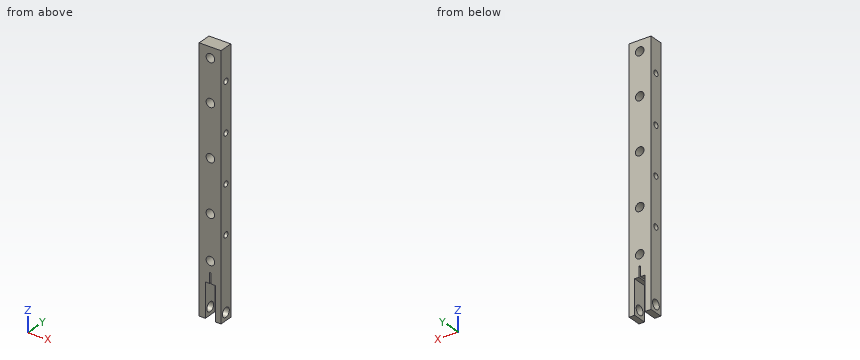
```python
from build123d import *

# Parameters (mm, degrees)
F1_DEPTH = 8
F3_D     = 5.5
F5_D     = 5
F7_D     = 3.3


with BuildPart() as f1:
    # F0 (on Front) → F1 (new body)
    with BuildSketch(Plane.XZ):
        Polygon((-6.6129033404, 0), (-3, 0), (-3, 20), (-0.5, 20), (-0.5, 26), (0.5, 26), (0.5, 20), (3, 20), (3, 0), (6.2258067564, 0), (6.2258067564, 150), (-6.6129033404, 150), align=None)
    extrude(amount=F1_DEPTH)

    # F3 (through all)
    with Locations(Plane(origin=(-6.6129033404, 0, 0), x_dir=(0, -1, 0), z_dir=(-1, 0, 0))):
        with Locations((4, 4.5417556539)):
            Hole(F3_D / 2)

    # F5 (through all)
    with Locations(Plane.XZ.offset(8)):
        with Locations((0, 32.4720963836), (0, 58.3593994379), (0, 88.90619874), (0, 119.1896349192), (0, 143.8203305006)):
            Hole(F5_D / 2)

    # F7 (through all)
    with Locations(Plane(origin=(-6.6129033404, 0, 0), x_dir=(0, -1, 0), z_dir=(-1, 0, 0))):
        with Locations((4, 131.3748806715), (4, 102.970726788), (4, 75), (4, 47.0387488604)):
            Hole(F7_D / 2)


solid = f1.part
```
Here's how the part is built. I have some questions about the finished solid (model axes, mm). Round coordinates to 2 decimals unless told otherwise and drop trailing zeros. Write each loop counter-clockwise with the first axis right and the second up, starting at its lowest first coordinate (ties: lowest second). Pieces come first, ordered by that corner, then holes.
Q1. If we section it at C-C on y = -4: Give the number of separate pieces and of enclosed holes in the cut face, plus the area to 3 significant figures.
Q2. Will this pin go through, and if not, where does the flat tip stop? P1, Ø0.8, axis at x = 2, y = -6, coming from the -Z side.
Q3. If we section it at B-B on x = 4.75: Write out the boundary of the cut face in (y, z), plus the area to 3 significant figures.
Q4. If we section it at A-A on z = 75: Write out the boundary of the cut face in (x, y), plus the area to 3 significant figures.
Q5. Please list where these lines run through material, in increasing order: probe 1 along Z at (x, y) = (0, -6); probe 2 along Z at (x, y) = (5.4, -4); probe 3 along Y at (x, z) = (2, 75.5).
Answer below:
1. separate pieces: 7
1. enclosed holes: 5
1. area: 1,490 mm2
2. P1: stops at z = 20
3. outline: (-8, 0) - (0, 0) - (0, 150) - (-8, 150) - close; hole circle Ø5.5 at (-4, 4.54); hole circle Ø3.3 at (-4, 47.04); hole circle Ø3.3 at (-4, 75); hole circle Ø3.3 at (-4, 102.97); hole circle Ø3.3 at (-4, 131.37)
3. area: 1,140 mm2
4. outline: (-6.61, -8) - (6.23, -8) - (6.23, -5.65) - (-6.61, -5.65) - close; (-6.61, -2.35) - (6.23, -2.35) - (6.23, 0) - (-6.61, 0) - close
4. area: 60.3 mm2
5. probe 1: z = 26 to 29.97, 34.97 to 55.86, 60.86 to 86.41, 91.41 to 116.69, 121.69 to 141.32, 146.32 to 150
5. probe 2: z = 0 to 1.79, 7.29 to 45.39, 48.69 to 73.35, 76.65 to 101.32, 104.62 to 129.72, 133.02 to 150
5. probe 3: y = -8 to -5.57, -2.43 to 0
